Geometry: final body of the model. Coordinates: model frame, mm. A direction names the side the tool comes from. Give positions to 0.01 mm unless a question says otherwise; leave off trailing zeros. Loops run counter-clockwise (first coordinate to the right, second up) from the corner with the lowest first, then second, coordinate; pieces in that order, holes last. Notation, with made-up numbers: (60.25, -10) -> (99.25, -10) arc R21 ccw to (99.25, 19) -> close; hole circle Ø10 at (-28, 32.25). An arc over 180 degrees is marked (long way). One line per question, with ' | ' between items. Start each with the question number.
Item 1: Mould query, pull axis Z, two halves, no side actions, for faces 1 (the flat face through (-13, -19.5, 6)), 2 (the flat face through (13.9, 13.7, 4.4)), 3 (the flat face through (0, 21.5, 6)), 4 (the flat face through (0, 0, 12)). Classes: released by +Z, released by -Z, zero draft, split by the parting line, or undercut.
Item 2: Section A-A on x = 0. Return loops of the section in (y, z).
Item 3: Set-up query: faces 5 (the flat face through (0, -4.9, 1)), 6 (the flat face through (15.545, -17.225, 8.093)), 7 (the flat face through (-13, 19.5, 6)), 8 (the flat face through (0, 0, 0)). Return all of +Z, -Z, +X, -X, +Y, -Y with unobstructed straight access to the full face (end or side cutting, diameter ignored); none if empty.
Item 4: Section C-C on z = 6.25. Return loops of the section in (x, y).
Item 5: Section D-D on y = -11. Return loops of the section in (x, z).
Item 6: Section B-B on z = 1.25. Return loops of the section in (x, y), then the cut area to 3 significant figures.
Item 7: Material intervals for line 1 along X through (y, z) = (15.5, 10); line 2 along Y through (x, z) = (12.5, 10.8); line 3 along Y through (x, z) = (0, 5.25), sorted ascending. Write a range as [from, to].
Autodesk Inventor part; units mm, degrees
ref_plane "YZ Plane" through (0, 0, 0) normal (1, 0, 0) x (0, 1, 0)
ref_plane "XZ Plane" through (0, 0, 0) normal (0, 1, 0) x (-1, 0, 0)
ref_plane "XY Plane" through (0, 0, 0) normal (0, 0, 1) x (1, 0, 0)
sketch "EsboçoBase" plane through (0, 0, 0) normal (0, 0, 1) x (1, 0, 0)
  line L0 (-12.5, 16.5) -> (12.5, 16.5) construction
  line L1 (12.5, 16.5) -> (12.5, -16.5) construction
  line L2 (12.5, -16.5) -> (-12.5, -16.5) construction
  line L3 (-12.5, -16.5) -> (-12.5, 16.5) construction
  line L4 (-12.5, 16.5) -> (12.5, -16.5) construction
  line L5 (12.5, 16.5) -> (-12.5, -16.5) construction
  line L6 (0, 16.5) -> (0, -16.5) construction
  line L7 (-12.5, 12.9) -> (12.5, 12.9) construction
  circle A0 centre (0, 9.9) radius 3
  line L8 (-12.5, 0) -> (12.5, 0) construction
  circle A1 centre (0, -9.9) radius 3
  line L9 (17.5, 21.5) -> (-17.5, 21.5)
  line L10 (-17.5, 21.5) -> (-17.5, -21.5)
  line L11 (-17.5, -21.5) -> (17.5, -21.5)
  line L12 (17.5, -21.5) -> (17.5, 21.5)
  line L13 (-2.8868, -4.9) -> (2.8868, -4.9)
  line L14 (2.8868, -4.9) -> (5.7735, -9.9)
  line L15 (5.7735, -9.9) -> (2.8868, -14.9)
  line L16 (2.8868, -14.9) -> (-2.8868, -14.9)
  line L17 (-2.8868, -14.9) -> (-5.7735, -9.9)
  line L18 (-5.7735, -9.9) -> (-2.8868, -4.9)
  line L19 (-2.8868, 4.9) -> (2.8868, 4.9)
  line L20 (2.8868, 4.9) -> (5.7735, 9.9)
  line L21 (5.7735, 9.9) -> (2.8868, 14.9)
  line L22 (2.8868, 14.9) -> (-2.8868, 14.9)
  line L23 (-2.8868, 14.9) -> (-5.7735, 9.9)
  line L24 (-5.7735, 9.9) -> (-2.8868, 4.9)
  circle A2 centre (12.5, -15.5) radius 2
  circle A3 centre (12.5, 15.5) radius 2
  circle A4 centre (-12.5, -15.5) radius 2
  circle A5 centre (-12.5, 15.5) radius 2
  line L25 (-14.5207, -12) -> (-10.4793, -12)
  line L26 (-10.4793, -12) -> (-8.4585, -15.5)
  line L27 (-8.4585, -15.5) -> (-10.4793, -19)
  line L28 (-10.4793, -19) -> (-14.5207, -19)
  line L29 (-14.5207, -19) -> (-16.5415, -15.5)
  line L30 (-16.5415, -15.5) -> (-14.5207, -12)
  point P0 (0, 0)
  point P1 (0, -9.9)
  dimension "d0" = 25
  dimension "d1" = 33
  dimension "d2" = 3.6
  dimension "d3" = 6
  dimension "d4" = 5
  dimension "d22" = 10
  dimension "d29" = 4
  dimension "d30" = 6
  dimension "d31" = 5
  dimension "d38" = 7
extrude "Adaptador" add sketch "EsboçoBase" along normal blind 12 contours A0 | A1 | L12 L11 L10 L9 | L13 L14 L15 L16 L17 L18 | L24 L23 L22 L21 L20 L19 | A2 | A3 | A4 | A5 | L25 L26 L27 L28 L29 L30
extrude "Furos" cut sketch "EsboçoBase" along normal blind 15 contours A0 | A1
thread "Thread1"
thread "Thread2"
sketch "Sketch5" plane through (-17.5, -21.5, 0) normal (-1, 0, 0) x (0, 0, 1)
  point P0 (0, 21.5)
extrude "Extrusion5" cut sketch "EsboçoBase" along normal blind 2 contours L13 L14 L15 L16 L17 L18 | L24 L23 L22 L21 L20 L19
sketch "PorcasLaterais" plane through (-17.5, -21.5, 0) normal (-1, 0, 0) x (0, 0, 1)
  line L0 (4.4, 2) -> (7.6, 2)
  line L1 (7.6, 2) -> (7.6, 10)
  line L2 (7.6, 10) -> (4.4, 10)
  line L3 (4.4, 10) -> (4.4, 2)
  line L4 (0, 0) -> (12, 0)
  line L5 (0, 43) -> (0, 0)
  line L6 (4.4, 6) -> (7.6, 6) construction
  line L7 (6, 2) -> (6, 10) construction
  line L8 (6, 0) -> (6, 43) construction
  line L9 (0, 6) -> (12, 6) construction
  line L10 (12, 43) -> (12, 0)
  point P0 (0, 21.5)
  dimension "d32" = 3.2
  dimension "d33" = 8
  dimension "d37" = 6
extrude "Extrusion6" cut sketch "PorcasLaterais" against normal blind 9.5
sketch "Sketch7" plane through (-17.5, -19.5, 7.6) normal (0, 0, -1) x (-1, 0, 0)
  line L0 (-9.0415, 4) -> (-7.0207, 0.5)
  line L1 (-7.0207, 7.5) -> (-9.0415, 4)
  line L2 (-2.9793, 7.5) -> (-7.0207, 7.5)
  line L3 (-0.9585, 4) -> (-2.9793, 7.5)
  line L4 (-2.9793, 0.5) -> (-0.9585, 4)
  line L5 (-7.0207, 0.5) -> (-2.9793, 0.5)
  point P0 (-17.5, 19.5)
extrude "Extrusion7" cut sketch "Sketch7" against normal blind 1
extrude "Extrusion8" cut sketch "EsboçoBase" along normal blind 12 contours A2 | A3 | A4 | A5
mirror "Mirror1" about plane through (0, 0, 0) normal (1, 0, 0) of "Extrusion6", "Extrusion7"
mirror "Mirror2" about plane through (0, 0, 0) normal (0, 1, 0) of "Extrusion7", "Extrusion6", "Mirror1"
properties part number "LoadCellBase"
Result sheet:
1) face 1: undercut | face 2: undercut | face 3: zero draft | face 4: released by +Z
2) outline: (-21.5, 0) -> (-14.9, 0) -> (-14.9, 2) -> (-12.9, 2) -> (-12.9, 12) -> (-21.5, 12) -> close; (-6.9, 2) -> (-4.9, 2) -> (-4.9, 0) -> (4.9, 0) -> (4.9, 2) -> (6.9, 2) -> (6.9, 12) -> (-6.9, 12) -> close; (12.9, 2) -> (14.9, 2) -> (14.9, 0) -> (21.5, 0) -> (21.5, 12) -> (12.9, 12) -> close
3) face 5: -Z | face 6: none | face 7: -X | face 8: -Z, +X, -X, +Y, -Y
4) outline: (-17.5, -21.5) -> (17.5, -21.5) -> (17.5, -19.5) -> (8, -19.5) -> (8, -11.5) -> (17.5, -11.5) -> (17.5, 11.5) -> (8, 11.5) -> (8, 19.5) -> (17.5, 19.5) -> (17.5, 21.5) -> (-17.5, 21.5) -> (-17.5, 19.5) -> (-8, 19.5) -> (-8, 11.5) -> (-17.5, 11.5) -> (-17.5, -11.5) -> (-8, -11.5) -> (-8, -19.5) -> (-17.5, -19.5) -> close; hole circle Ø6 at (0, -9.9); hole circle Ø6 at (0, 9.9)
5) outline: (-17.5, 0) -> (-5.14, 0) -> (-5.14, 2) -> (-2.79, 2) -> (-2.79, 12) -> (-17.5, 12) -> close; (2.79, 2) -> (5.14, 2) -> (5.14, 0) -> (17.5, 0) -> (17.5, 12) -> (2.79, 12) -> close
6) outline: (-17.5, -21.5) -> (17.5, -21.5) -> (17.5, 21.5) -> (-17.5, 21.5) -> close; hole circle Ø4 at (-12.5, -15.5); hole circle Ø4 at (-12.5, 15.5); hole (-5.77, -9.9) -> (-2.89, -14.9) -> (2.89, -14.9) -> (5.77, -9.9) -> (2.89, -4.9) -> (-2.89, -4.9) -> close; hole (-5.77, 9.9) -> (-2.89, 4.9) -> (2.89, 4.9) -> (5.77, 9.9) -> (2.89, 14.9) -> (-2.89, 14.9) -> close; hole circle Ø4 at (12.5, -15.5); hole circle Ø4 at (12.5, 15.5) | area: 1,280 mm²
7) line 1: x = [-17.5, -14.5], [-10.5, 10.5], [14.5, 17.5] | line 2: y = [-21.5, -17.5], [-13.5, 13.5], [17.5, 21.5] | line 3: y = [-21.5, -12.9], [-6.9, 6.9], [12.9, 21.5]
